```python
from build123d import *

# Parameters (mm, degrees)
SKETCH2_R          = 1.35
CUT_EXTRUDE1_DEPTH = 71.865707448
SKETCH4_R          = 25
CUT_EXTRUDE2_DEPTH = 71.865707448


with BuildPart() as part:
    # Sketch1 → Revolve1 (revolve)
    with BuildSketch(Plane.XY, mode=Mode.PRIVATE) as revolve1_sk:
        with BuildLine():
            Line((0, 0.315015275), (-47.48443706, 0.315015275))
            ThreePointArc((-47.48443706, 0.315015275), (-48.325204531, 1.887561025), (-50, 2.499811149))
            Line((-50, 2.499811149), (-50, 4.999937053))
            Line((-50, 4.999937053), (0, 4.999937053))
            Line((0, 4.999937053), (0, 0.315015275))
        make_face()
    revolve(revolve1_sk.sketch.rotate(Axis((0, 0.315015275, 0), (0, 1, 0)), 270), axis=Axis((0, 0.315015275, 0), (0, 1, 0)))

    # Sketch2 → Cut-Extrude1 (cut, through all)
    with BuildSketch(Plane(origin=(0, 4.999937053, 0), x_dir=(1, 0, 0), z_dir=(0, 1, 0))):
        with Locations(Location((0, 32.5, 0), (0, 0, 270))):
            Circle(SKETCH2_R)
        with Locations(Location((22.980970389, 22.980970389, 0), (0, 0, 270))):
            Circle(SKETCH2_R)
        with Locations(Location((32.5, 0, 0), (0, 0, 270))):
            Circle(SKETCH2_R)
        with Locations(Location((22.980970389, -22.980970389, 0), (0, 0, 270))):
            Circle(SKETCH2_R)
        with Locations(Location((0, -32.5, 0), (0, 0, 270))):
            Circle(SKETCH2_R)
        with Locations(Location((-22.980970389, -22.980970389, 0), (0, 0, 270))):
            Circle(SKETCH2_R)
        with Locations(Location((-32.5, 0, 0), (0, 0, 270))):
            Circle(SKETCH2_R)
        with Locations(Location((-22.980970389, 22.980970389, 0), (0, 0, 270))):
            Circle(SKETCH2_R)
    extrude(amount=-CUT_EXTRUDE1_DEPTH, mode=Mode.SUBTRACT)

    # Sketch4 → Cut-Extrude2 (cut, through all)
    with BuildSketch(Plane.XZ.offset(-0.315015275)):
        with Locations(Location((0, 0, 0), (0, 0, 270))):
            Circle(SKETCH4_R)
    extrude(amount=-CUT_EXTRUDE2_DEPTH, mode=Mode.SUBTRACT)


solid = part.part
```
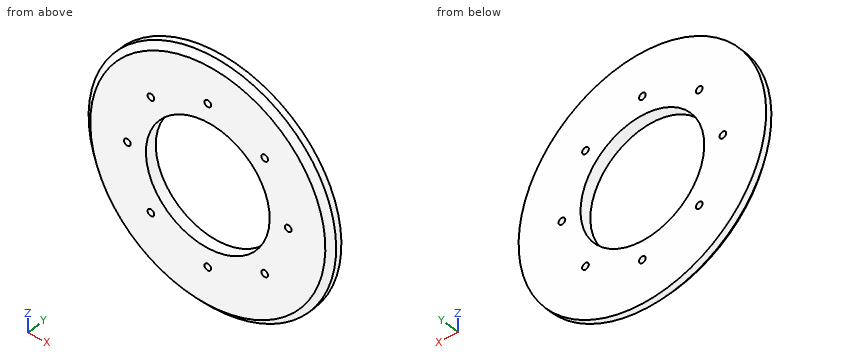
CAD build for the part. Positions are in the model's coordinates, mm. Round coordinates to 2 decimals unless told otherwise and drop trailing zeros. Order: outer loops, then holes, each group sorted by start corner. A loop starts at its lowest first (then second) coordinate and runs counter-clockwise, first axis right, second up.
Q1. Slice it at A-A (x = 0). Write the cut outline in (y, z).
Q2. Drop flat-ended pins along their axis: pin 1 (1.5 mm diameter, centred on x = 10.5, y = 4, fed in from -Z); pin 2 (1.5 mm diameter, centred on x = -11, y = 3.5, fed in from -Z). Give the stop position or say it passes through.
Q3. Slice it at B-B (y = 1.1). State how many separate pieces and enclosed holes the cut face has, and give its area (3 significant figures).
Q4. Wall check: L1, parallel to X at y = 2.7, z = 0; L2, parallel to X at y = 1.6, z = 0; L3, parallel to X at y = 4.05, z = 6.5. Give the ranges that are in metal, low to high.
Results below:
1. outline: (0.32, -47.48) arc R2.5 cw to (2.5, -50) - (5, -50) - (5, -33.85) - (0.32, -33.85) - close; (0.32, -31.15) - (5, -31.15) - (5, -25) - (0.32, -25) - close; (0.32, 25) - (5, 25) - (5, 31.15) - (0.32, 31.15) - close; (0.32, 33.85) - (5, 33.85) - (5, 50) - (2.5, 50) arc R2.5 cw to (0.32, 47.48) - close
2. pin 1: stops at z = -49.04
2. pin 2: stops at z = -48.94
3. separate pieces: 1
3. enclosed holes: 9
3. area: 5,140 mm2
4. L1: x = -50 to -33.85, -31.15 to -25, 25 to 31.15, 33.85 to 50
4. L2: x = -48.04 to -33.85, -31.15 to -25, 25 to 31.15, 33.85 to 48.04
4. L3: x = -49.58 to -24.14, 24.14 to 49.58
